Source: CAD feature listing. Evaluate the final solid. Frame: model axes, mm. A direction names the side the tool comes from. Round coordinates to 2 decimals unless told otherwise and drop trailing zeros. Write each loop counter-clockwise with the first axis right and the second up, starting at its lowest first coordinate (ties: lowest second). Pieces come first, ordered by that corner, then holes. Notation, with made-up numbers: (-32.75, 78.25) -> (-23.75, 78.25) arc R31 cw to (-23.75, 108.25) -> close; hole circle Ø2 at (45, -28). An arc over 180 degrees is marked (long way). Put each result on its own line as item: value.
```python
from build123d import *

# Parameters (mm, degrees)
F0_R     = 2.2225
F0_R_2   = 3.556
F0_R_3   = 2.54
F1_DEPTH = 6.35


with BuildPart() as f1:
    # F0 (on Top) → F1 (new body)
    with BuildSketch(Plane.XY):
        with BuildLine():
            Line((45.72, 50.8), (-45.72, 50.8))
            ThreePointArc((-45.72, 50.8), (-49.312102, 49.312102), (-50.8, 45.72))
            Line((-50.8, 45.72), (-50.8, -45.72))
            ThreePointArc((-50.8, -45.72), (-49.312102, -49.312102), (-45.72, -50.8))
            Line((-45.72, -50.8), (45.72, -50.8))
            ThreePointArc((45.72, -50.8), (49.312102, -49.312102), (50.8, -45.72))
            Line((50.8, -45.72), (50.8, 45.72))
            ThreePointArc((50.8, 45.72), (49.312102, 49.312102), (45.72, 50.8))
        make_face()
        with Locations((-46.0375, -46.0375)):
            Circle(F0_R, mode=Mode.SUBTRACT)
        with BuildLine():
            ThreePointArc((-9.939316, -24.3), (10, -25.4), (-9.939316, -26.5))
            Line((-9.939316, -26.5), (-11.1, -26.5))
            Line((-11.1, -26.5), (-11.1, -25.4))
            Line((-11.1, -25.4), (-11.1, -24.3))
            Line((-11.1, -24.3), (-9.939316, -24.3))
        make_face(mode=Mode.SUBTRACT)
        Circle(F0_R_2, mode=Mode.SUBTRACT)
        with Locations((46.0375, -46.0375)):
            Circle(F0_R, mode=Mode.SUBTRACT)
        with Locations((-21.997045, 12.7)):
            Circle(F0_R_3, mode=Mode.SUBTRACT)
        with Locations((-8.687312, 23.868193)):
            Circle(F0_R_3, mode=Mode.SUBTRACT)
        with Locations((-46.0375, 46.0375)):
            Circle(F0_R, mode=Mode.SUBTRACT)
        with Locations((8.687312, 23.868193)):
            Circle(F0_R_3, mode=Mode.SUBTRACT)
        with Locations((21.997045, 12.7)):
            Circle(F0_R_3, mode=Mode.SUBTRACT)
        with Locations((46.0375, 46.0375)):
            Circle(F0_R, mode=Mode.SUBTRACT)
    extrude(amount=F1_DEPTH)


solid = f1.part
```
Q1. Pin query (flat end, axial travel): pin 1 (3 mm diameter, centred on x = 8.69, y = 23.87, fed in from +Z). Return the tip coordinate at first contact, or that it passes through.
Ans:
pin 1: passes through
Q2. Cut plane D-D on z = 1.25. Give the number of separate pieces and of enclosed holes in the cut face, and give its area (3 significant figures).
Ans:
separate pieces: 1
enclosed holes: 10
area: 9,800 mm^2
Q3. Material intervals for line 1 (X direction, y = 23.5, z = 0.5); line 2 (Y direction, x = 0, z = 4.5); line 3 (X direction, y = 13, z = 3), sorted ascending. Write a range as [from, to].
Ans:
line 1: x = [-50.8, -11.2], [-6.17, 6.17], [11.2, 50.8]
line 2: y = [-50.8, -35.4], [-15.4, -3.56], [3.56, 50.8]
line 3: x = [-50.8, -24.52], [-19.47, 19.47], [24.52, 50.8]
Q4. Cut plane C-C on y = 12.7. Output: boundary loops of the cut face in (x, z), and give its area (3 significant figures).
Ans:
outline: (-50.8, 0) -> (-24.54, 0) -> (-24.54, 6.35) -> (-50.8, 6.35) -> close; (-19.46, 0) -> (19.46, 0) -> (19.46, 6.35) -> (-19.46, 6.35) -> close; (24.54, 0) -> (50.8, 0) -> (50.8, 6.35) -> (24.54, 6.35) -> close
area: 581 mm^2
Q5. Cut plane B-B on y = 0. Output: boundary loops of the cut face in (x, z).
Ans:
outline: (-50.8, 0) -> (-3.56, 0) -> (-3.56, 6.35) -> (-50.8, 6.35) -> close; (3.56, 0) -> (50.8, 0) -> (50.8, 6.35) -> (3.56, 6.35) -> close
Q6. Cut plane A-A on x = 0. Output: boundary loops of the cut face in (y, z), and give its area (3 significant figures).
Ans:
outline: (-50.8, 0) -> (-35.4, 0) -> (-35.4, 6.35) -> (-50.8, 6.35) -> close; (-15.4, 0) -> (-3.56, 0) -> (-3.56, 6.35) -> (-15.4, 6.35) -> close; (3.56, 0) -> (50.8, 0) -> (50.8, 6.35) -> (3.56, 6.35) -> close
area: 473 mm^2
Q7. Draft query along Y for faces 1 (the cylindrical face through (-49.272, 49.351, 3.131)), 2 (the cylindrical face through (-9.018, 26.387, 3.131)), 3 (the flat face through (11, 1, 6.35)). Return one class per face: +Y half, -Y half, draft (parallel to the pull), parting line (faces both ways), or undercut.
Ans:
face 1: +Y half
face 2: undercut
face 3: draft
Q8. Reachability of faces 4 (the flat face through (-1, -50.8, 3)), 5 (the flat face through (-11.1, -25, 3)) from +Z, -Z, +X, -X, +Y, -Y: full face, straight path, thin tool, end or side. Return the list, or none.
Ans:
face 4: +Z, -Z, +X, -X, -Y
face 5: +Z, -Z
